The drawing under review shows one solid part. Ordinate dimensions are in mm from its lowest x, y, z. A direction names the side the tool comes from. Give positions to 0.01 mm unless a question says otherwise; leave off trailing zeros. Write each loop counter-clockwise with the first axis right and the second up, starting at its lowest first coordinate (ties: lowest second). Pieces come first, ordered by that corner, then holes. Notation, with made-up numbers: M 46.25,-28 L 53.25,-28 A33 ccw 53.25,3 Z; hole C 10,38 d2. An arc over 180 degrees is marked long. Answer as a JSON object with one key per item and string values. Group by question number.
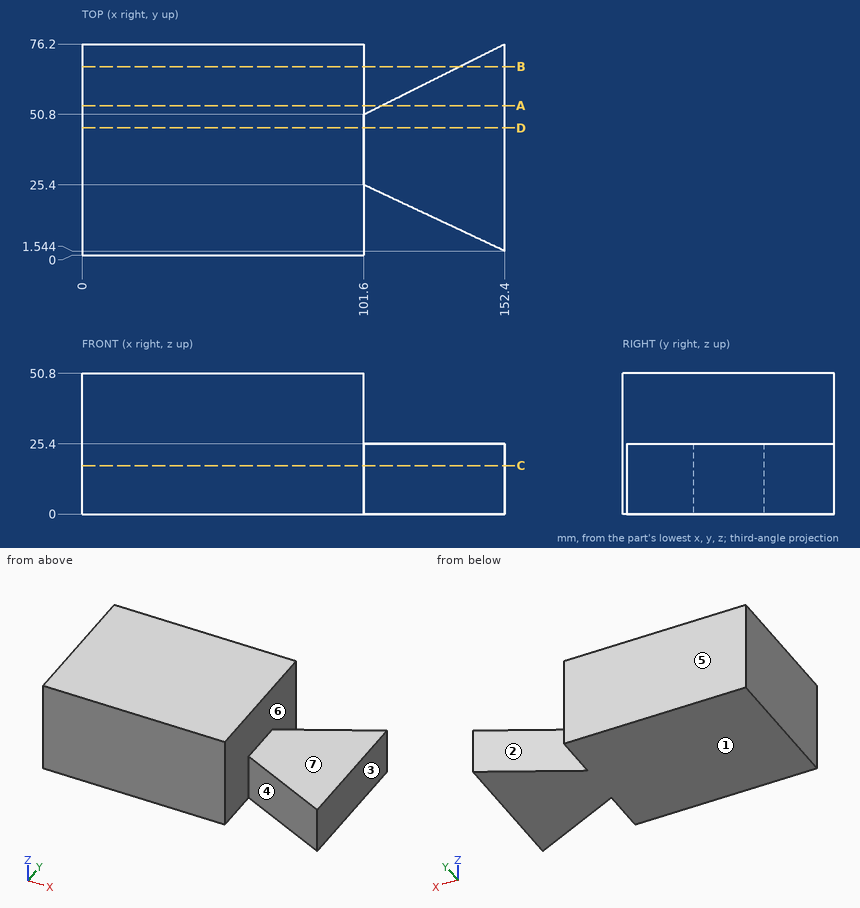
Item 1: Consider section C-C (z = 17.5). Give the boundary of the cut face in (x, y) (1 decimal), plus the area to 3 significant figures.
Item 2: Machinability: for the marked faces 5, 6 and 7, which of the approach directions +Z, -Z, +X, -X, +Y, -Y give a long, thin tool a straight path to every point of the face, cutting with its end or side? Answer none if there is none.
Item 3: Draft analysis for pull direction X (two halves, no side actions). For the marked faces 1, 2, 3 and 4, state which applies: released by +X, released by -X, zero draft, split by the parting line, or undercut.
Item 4: Consider section B-B (y = 68). Give the boundary of the cut face in (x, z).
Item 5: Consider section A-A (y = 54). Give the boundary of the cut face in (x, z), plus the area to 3 significant figures.
Item 6: Consider section D-D (y = 46). Give the boundary of the cut face in (x, z), plus the area to 3 significant figures.
Item 7: Insertion check: P1, Ø10, axis at x = 109.5, z = 20.5, coming from the +Y side. The pin has a flat end and moves straight along its axis. Give the tip position at first contact, or say it passes through.
Item 8: To check wall thickness, follow probe 1 along Z at (x, y) = (136.5, 65); probe 2 along X at (y, z) = (51, 13); probe 3 along X at (y, z) = (5, 20) (1 decimal). State the ranges of each line that lie inside material, in increasing order.
Result set:
{
 "1": {"outline": "M 0,0 L 101.6,0 L 101.6,25.4 L 152.4,1.5 L 152.4,76.2 L 101.6,50.8 L 101.6,76.2 L 0,76.2 Z", "area": "10,300 mm^2"},
 "2": {"face 5": "+Z, -Z, +X, -X, +Y", "face 6": "+Z", "face 7": "+Z, +X, +Y, -Y"},
 "3": {"face 1": "zero draft", "face 2": "undercut", "face 3": "released by +X", "face 4": "undercut"},
 "4": {"outline": "M 0,0 L 101.6,0 L 101.6,50.8 L 0,50.8 Z; M 136,0 L 152.4,0 L 152.4,25.4 L 136,25.4 Z"},
 "5": {"outline": "M 0,0 L 101.6,0 L 101.6,50.8 L 0,50.8 Z; M 108,0 L 152.4,0 L 152.4,25.4 L 108,25.4 Z", "area": "6,290 mm^2"},
 "6": {"outline": "M 0,0 L 152.4,0 L 152.4,25.4 L 101.6,25.4 L 101.6,50.8 L 0,50.8 Z", "area": "6,450 mm^2"},
 "7": {"P1": "stops at y = 57.25"},
 "8": {"probe 1": "z = 0 to 25.4", "probe 2": "x = 0 to 101.6, 102 to 152.4", "probe 3": "x = 0 to 101.6, 145 to 152.4"}
}
